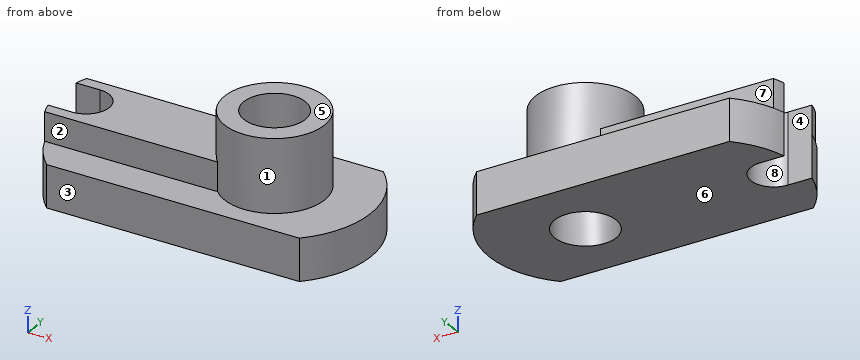
from build123d import *

# Parameters (mm, degrees)
BOSS_EXTRUDE1_DEPTH = 11
BOSS_EXTRUDE2_DEPTH = 7.5
SKETCH2_3_R         = 13
SKETCH2_3_R_2       = 8
BOSS_EXTRUDE3_DEPTH = 19
SKETCH8_R           = 8
CUT_EXTRUDE1_DEPTH  = 19


with BuildPart() as part:
    # Sketch1 → Boss-Extrude1 (new body)
    with BuildSketch(Plane.XY):
        with BuildLine():
            Line((-32.849351573, -18), (32.849351573, -18))
            ThreePointArc((32.849351573, -18), (40.5, 0), (32.849351573, 18))
            Line((32.849351573, 18), (-32.849351573, 18))
            ThreePointArc((-32.849351573, 18), (-37.157065859, 12.488854966), (-39.769322199, 6))
            Line((-39.769322199, 6), (-33.5, 6))
            ThreePointArc((-33.5, 6), (-27.5, 0), (-33.5, -6))
            Line((-33.5, -6), (-39.769322199, -6))
            ThreePointArc((-39.769322199, -6), (-37.157065859, -12.488854966), (-32.849351573, -18))
        make_face()
    extrude(amount=-BOSS_EXTRUDE1_DEPTH)

    # Sketch2 → Boss-Extrude2 (add)
    with BuildSketch(Plane.XY):
        with BuildLine():
            ThreePointArc((-39.769322199, -6), (-39.343793753, -7.514885194), (-38.823807579, -9))
            Line((-38.823807579, -9), (6.11916848, -9))
            ThreePointArc((6.11916848, -9), (2.5, 0), (6.11916848, 9))
            Line((6.11916848, 9), (-38.823807579, 9))
            ThreePointArc((-38.823807579, 9), (-39.343793753, 7.514885194), (-39.769322199, 6))
            Line((-39.769322199, 6), (-33.5, 6))
            ThreePointArc((-33.5, 6), (-27.5, 0), (-33.5, -6))
            Line((-33.5, -6), (-39.769322199, -6))
        make_face()
    extrude(amount=BOSS_EXTRUDE2_DEPTH)

    # Sketch2<3> → Boss-Extrude3 (add)
    with BuildSketch(Plane.XY):
        with Locations((15.5, 0)):
            Circle(SKETCH2_3_R)
        with Locations((15.5, 0)):
            Circle(SKETCH2_3_R_2, mode=Mode.SUBTRACT)
    extrude(amount=BOSS_EXTRUDE3_DEPTH)

    # Sketch8 → Cut-Extrude1 (cut)
    with BuildSketch(Plane.XY):
        with Locations((15.5, 0)):
            Circle(SKETCH8_R)
    extrude(amount=-CUT_EXTRUDE1_DEPTH, mode=Mode.SUBTRACT)


solid = part.part
Here's how the part is built. I have some questions about the finished solid (model axes, mm). Face numbers are marked on the shaded views. A direction names the side the tool comes from. Coordinates: 2 decimals unless noted, no trailing zeros. Order: outer loops, then holes, each group sorted by start corner. A loop starts at its lowest first (then second) coordinate and runs counter-clockwise, first axis right, second up.
Item 1: For P1, Ø4, axis at x = 15, z = 10.5, coming from the +Y side; P2, Ø8, axis at x = -24.5, z = 5.5, coming from the +Y side; P3, Ø11, axis at x = -13, y = -7, coming from the +Z side, each with a flat end and sliding along its axis, tell me the tip position at first contact or that it passes through.
Result sheet:
P1: stops at y = 13
P2: stops at y = 9
P3: stops at z = 7.5
Item 2: For the marked faces 1, 2, 3, 4 and 5, which set-ups out of +Z, -Z, +X, -X, +Y, -Y let a thin tool reach every point of the face, with its end or its side?
Result sheet:
face 1: +Z
face 2: +Z, -X, -Y
face 3: +Z, -Z, +X, -X, -Y
face 4: +Z, -Z, -X
face 5: +Z, +X, -X, +Y, -Y
Item 3: I need wall thicknesses on line 1 (Y direction, x = 15.5, z = -4); line 2 (Y direction, x = 15.5, z = 5.25); line 3 (Z direction, x = -10.5, y = 12.5). Which ranges of each line are inside material? Lowest first, please.
Result sheet:
line 1: y = -18 to -8, 8 to 18
line 2: y = -13 to -8, 8 to 13
line 3: z = -11 to 0
Item 4: If we section it at B-B on y = 0: List the corners of the cut face in (x, z) for me.
Result sheet:
outline: (-27.5, -11) - (7.5, -11) - (7.5, 19) - (2.5, 19) - (2.5, 7.5) - (-27.5, 7.5) - close; (23.5, -11) - (40.5, -11) - (40.5, 0) - (28.5, 0) - (28.5, 19) - (23.5, 19) - close
Item 5: If we section it at C-C on z = 3.75: List the corners of the cut face in (x, y) for me, plus the area to 3 significant figures.
Result sheet:
outline: (-39.77, -6) arc R25 ccw to (-38.82, -9) - (6.12, -9) arc R13 ccw (long way) to (6.12, 9) - (-38.82, 9) arc R25 ccw to (-39.77, 6) - (-33.5, 6) arc R6 cw to (-33.5, -6) - close; hole circle Ø16 at (15.5, 0)
area: 977 mm2
Item 6: If we section it at D-D on x = -6: List the corners of the cut face in (y, z) for me.
Result sheet:
outline: (-18, -11) - (18, -11) - (18, 0) - (9, 0) - (9, 7.5) - (-9, 7.5) - (-9, 0) - (-18, 0) - close
Item 7: If we mould it in two halves opening along Y, with no side actions, what happens to the marked faces 6, 7 and 8? For each: +Y half, -Y half, draft (parallel to the pull), parting line (faces both ways), or undercut.
Result sheet:
face 6: draft
face 7: +Y half
face 8: undercut
Item 8: If we section it at A-A on x = 15.5: List the corners of the cut face in (y, z) for me.
Result sheet:
outline: (-18, -11) - (-8, -11) - (-8, 19) - (-13, 19) - (-13, 0) - (-18, 0) - close; (8, -11) - (18, -11) - (18, 0) - (13, 0) - (13, 19) - (8, 19) - close
